Part print with two shaded views. Sizes in mm from the minimum x, y, z corner. A direction names the side the tool comes from. Coordinates: 2 decimals unless noted, no trailing zeros. Order: outer loops, then holes, each group sorted by start corner. A loop starts at its lowest first (then second) coordinate and runs counter-clockwise, first axis right, second up.
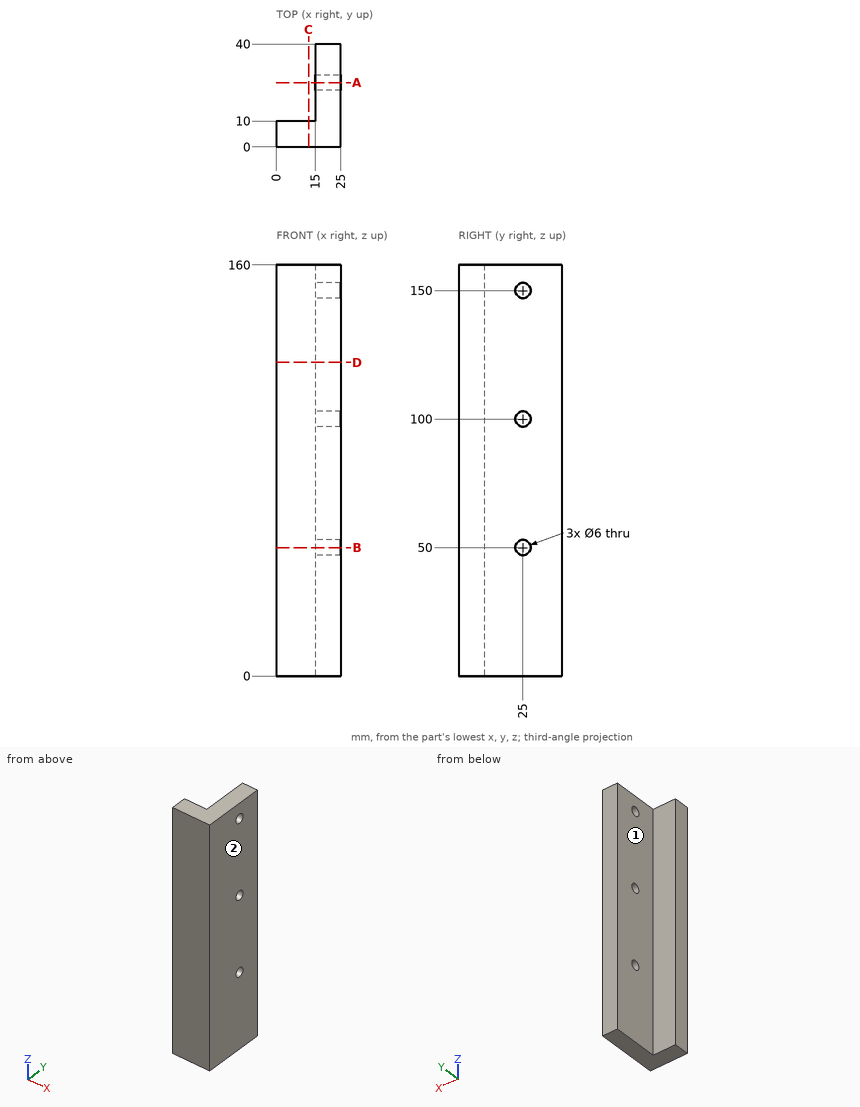
Q1. Cut at C-C on x = 12.5. Write the cut outline in (y, z).
Results list:
outline: (0, 0) - (10, 0) - (10, 160) - (0, 160) - close
Q2. Wall check: line 1 along Z through (x, y) = (23.25, 25); line 2 along Y through (x, z) = (17.5, 100); line 3 along X through (y, z) = (33, 112.5). Give the ranges that are in metal, low to high.
Results list:
line 1: z = 0 to 47, 53 to 97, 103 to 147, 153 to 160
line 2: y = 0 to 22, 28 to 40
line 3: x = 15 to 25
Q3. Cut at A-A on y = 25. Write the cut outline in (x, z), and give its area (3 significant figures).
Results list:
outline: (15, 0) - (25, 0) - (25, 47) - (15, 47) - close; (15, 53) - (25, 53) - (25, 97) - (15, 97) - close; (15, 103) - (25, 103) - (25, 147) - (15, 147) - close; (15, 153) - (25, 153) - (25, 160) - (15, 160) - close
area: 1,420 mm2
Q4. Which spindle directions (+Z, -Z, +X, -X, +Y, -Y) get a long thin tool onto all of the face, cutting with end or side? Do the marked faces 1 and 2. Say none if no direction does.
Results list:
face 1: +Z, -Z, -X, +Y
face 2: +Z, -Z, +X, +Y, -Y
Q5. Cut at D-D on z = 122. Write the cut outline in (x, y), and give its area (3 significant figures).
Results list:
outline: (0, 0) - (25, 0) - (25, 40) - (15, 40) - (15, 10) - (0, 10) - close
area: 550 mm2
Q6. Pin check, flat tips, straight feed: pin 1 Ø3.5 at (y, z) = (25, 50) entering from -X; pin 2 Ø9 at (y, z) = (31.5, 61.5) entering from -X; pin 3 Ø4.5 at (x, z) = (5, 83) entering from +Y. Stop position of each tip, or through.
Results list:
pin 1: passes through
pin 2: stops at x = 15
pin 3: stops at y = 10
Q7. Cut at B-B on z = 50. Write the cut outline in (x, y).
Results list:
outline: (0, 0) - (25, 0) - (25, 22) - (15, 22) - (15, 10) - (0, 10) - close; (15, 28) - (25, 28) - (25, 40) - (15, 40) - close
